from build123d import *

# Parameters (mm, degrees)
SKETCH2_W           = 17.78
SKETCH2_H           = 25.4
BOSS_EXTRUDE1_DEPTH = 6.35
SKETCH3_R           = 1.326085058
SKETCH3_R_2         = 1.159154329
CUT_EXTRUDE2_DEPTH  = 3.81
CUT_EXTRUDE3_REACH  = 19.78
SKETCH4_W           = 22.86
SKETCH4_H           = 3.81


with BuildPart() as part:
    # Sketch2 → Boss-Extrude1 (new body)
    with BuildSketch(Plane(origin=(0, 0, 0), x_dir=(1, 0, 0), z_dir=(0, 1, 0))):
        with Locations((8.89, 12.7)):
            Rectangle(SKETCH2_W, SKETCH2_H)
    extrude(amount=BOSS_EXTRUDE1_DEPTH)

    # Sketch3 → Cut-Extrude2 (cut)
    with BuildSketch(Plane(origin=(0, 6.35, 0), x_dir=(1, 0, 0), z_dir=(0, 1, 0))):
        with Locations((2.54, 7.552937487)):
            Circle(SKETCH3_R)
        with Locations((15.24, 7.552937487)):
            Circle(SKETCH3_R_2)
    extrude(amount=-CUT_EXTRUDE2_DEPTH, mode=Mode.SUBTRACT)

    # Sketch4 → Cut-Extrude3 (cut, up to next)
    with BuildSketch(Plane(origin=(17.78, 0, 0), x_dir=(0, 0, -1), z_dir=(1, 0, 0)), mode=Mode.PRIVATE) as cut_extrude3_sk1:
        with Locations((12.7, 3.175)):
            Rectangle(SKETCH4_W, SKETCH4_H)
    cut_extrude3_tool1 = extrude(cut_extrude3_sk1.sketch, amount=-CUT_EXTRUDE3_REACH, mode=Mode.PRIVATE) & part.part
    add(cut_extrude3_tool1.solids().sort_by_distance((17.78, 3.175, -12.7))[0], mode=Mode.SUBTRACT)


solid = part.part
The listing builds one solid part. Answer for the finished solid, in the listing's coordinates (mm). A direction names the side the tool comes from. Coordinates: 2 decimals unless noted, no trailing zeros. Write each loop counter-clockwise with the first axis right and the second up, starting at its lowest first coordinate (ties: lowest second). Pieces come first, ordered by that corner, then holes. Notation, with made-up numbers: M 3,25 L 39,25 A19 cw 39,53 Z; hole C 81.25,36 d10. An arc over 180 degrees is marked long. Put each result on its own line as item: value. Start each with the question number.
1. A cutting plane is placed at C-C on x = 2.54. Write down the section's boundary in (y, z).
2. Consider line 1 (Y direction, x = 4.5, z = -13); line 2 (Z direction, x = 15.24, y = 5.7); line 3 (Z direction, x = 2, y = 4.25). Determine where each line is inside the solid, lowest interval first. Write a range as from..to.
3. Which of the six approach directions +Z, -Z, +X, -X, +Y, -Y give full straight-line access (tool end or side, diameter ignored) to faces 1 (the flat face through (0, 1, -13)), 2 (the flat face through (9, 5.08, -13)), 3 (the cylindrical face through (2.37, 5.72, -8.87))?
4. For a pull along Z with two mould halves and no side action, classify faces 4 (the flat face through (9, 0, -13)), 5 (the flat face through (9, 1.27, -13)), 6 (the cylindrical face through (14.32, 5.72, -6.85)), 7 (the flat face through (9, 3, 0)) as pulls with the +Z half, pulls with the -Z half, needs draft (parallel to the pull), parting line crosses it, or undercut.
5. A cutting plane is placed at B-B on z = -8. Write down the section's boundary in (x, y).
6. A flat-ended cylindrical pin translates along its axis: P1, Ø1.4, axis at x = 15.24, z = -7.55, coming from the +Y side. Find the tip coordinate at first contact, or state that the pin passes through.
7. A cutting plane is placed at A-A on y = 4.75. Write down the section's boundary in (x, z), then the cut area to 3 significant figures.
8. A cutting plane is placed at D-D on x = 6.25. Write down the section's boundary in (y, z).
Resolved:
1. outline: M 0,-25.4 L 6.35,-25.4 L 6.35,-8.88 L 5.08,-8.88 L 5.08,-24.13 L 1.27,-24.13 L 1.27,-1.27 L 5.08,-1.27 L 5.08,-6.23 L 6.35,-6.23 L 6.35,0 L 0,0 Z
2. line 1: y = 0..1.27, 5.08..6.35
2. line 2: z = -25.4..-8.71, -6.39..0
2. line 3: z = -25.4..-24.13, -1.27..0
3. face 1: +Z, -Z, -X, +Y, -Y
3. face 2: +X, -X
3. face 3: +Y
4. face 4: needs draft
4. face 5: undercut
4. face 6: undercut
4. face 7: pulls with the +Z half
5. outline: M 0,0 L 17.78,0 L 17.78,1.27 L 0,1.27 Z; M 0,5.08 L 1.29,5.08 L 1.29,6.35 L 0,6.35 Z; M 3.79,5.08 L 14.17,5.08 L 14.17,6.35 L 3.79,6.35 Z; M 16.31,5.08 L 17.78,5.08 L 17.78,6.35 L 16.31,6.35 Z
6. P1: stops at y = 1.27
7. outline: M 0,-25.4 L 17.78,-25.4 L 17.78,-24.13 L 0,-24.13 Z; M 0,-1.27 L 17.78,-1.27 L 17.78,0 L 0,0 Z
7. area: 45.2 mm2
8. outline: M 0,-25.4 L 6.35,-25.4 L 6.35,0 L 0,0 Z; hole M 1.27,-24.13 L 5.08,-24.13 L 5.08,-1.27 L 1.27,-1.27 Z
